Read the model definition and answer for the solid it produces. Units are mm, in the model's axes. A direction names the side the tool comes from. Coordinates: 2 decimals unless noted, no trailing zeros. Write each loop counter-clockwise with the first axis right and the second up, starting at its lowest first coordinate (ties: lowest second). Pieces come first, ordered by that corner, then holes. Notation, with made-up numbers: (11, -10) -> (53, -10) arc R36 ccw to (53, 24) -> close; hole circle Ø5 at (-13, -20). An arc over 180 degrees is marked (long way). One line per item, written item: value. Start each with the question number.
1. For faces 1 (the flat face through (3, -22, -76.2)), 2 (the flat face through (3, -29, 38.1)), 3 (the flat face through (3, 0, 73)), 4 (the flat face through (3, -6, -69.85)), 5 (the flat face through (3, -9, 59.382)), determine the directions among +Z, -Z, +X, -X, +Y, -Y from which every point of the face is accessible in a straight line to the end or side of a thin tool.
2. Find section A-A, the plane y = -4. Write down the section's boundary in (x, z), and give its area (3 significant figures).
3. Find section B-B, the plane z = -2.5. Write down the section's boundary in (x, y), and give its area (3 significant figures).
4. Find section C-C, the plane y = -27.5. Write down the section's boundary in (x, z).
5. Find section D-D, the plane y = 8.5. Write down the section's boundary in (x, z).
6. For a pull along Z with two mould halves and no side action, classify faces 6 (the flat face through (6.35, 10, 1)), 7 (the flat face through (3, 19, 76.2)), 8 (the flat face through (3, -29, -38.1)), 9 (the flat face through (3, -21.293, 3)) as pulls with the +Z half, pulls with the -Z half, needs draft (parallel to the pull), parting line crosses it, or undercut.
7. Given P1, Ø1.9, axis at x = 4, y = 22, coming from the -Z side; P2, Ø3, axis at x = 3, y = 7.5, coming from the +Z side; P3, Ø3, axis at x = 1.5, z = 45, coming from the -Y side, each flat-ended and moving along its own axis, determine where each tip first touches the part or whether it passes through.
8. Consider line 1 along Z through (x, y) = (6.25, -27); line 2 along Z through (x, y) = (3, 21); line 3 along Y through (x, z) = (2.5, 32.5). Determine where each line is inside the solid, lowest interval first.
```python
from build123d import *

# Parameters (mm, degrees)
SKETCH1_W           = 114.3
SKETCH1_H           = 25.4
BOSS_EXTRUDE1_DEPTH = 6.35
SKETCH1_4_W         = 6.35
SKETCH1_4_H         = 6.35
BOSS_EXTRUDE2_DEPTH = 6.35


with BuildPart() as part:
    # Sketch1 → Boss-Extrude1 (new body)
    with BuildSketch(Plane(origin=(0, 0, 0), x_dir=(0, 0, -1), z_dir=(1, 0, 0))):
        Polygon((-76.2, 25.4), (-76.2, 12.7), (-69.85, 12.7), (-69.85, 0), (-76.2, 0), (-76.2, -12.7), (-69.85, -12.7), (-69.85, -31.75), (-63.5, -31.75), (-63.5, -25.4), (-38.1, -25.4), (-38.1, -31.75), (-31.75, -31.75), (-31.75, -25.4), (31.75, -25.4), (31.75, -31.75), (38.1, -31.75), (38.1, -25.4), (63.5, -25.4), (63.5, -31.75), (69.85, -31.75), (69.85, -25.4), (76.2, -25.4), (76.2, -12.7), (69.85, -12.7), (69.85, 0), (76.2, 0), (76.2, 12.7), (69.85, 12.7), (69.85, 25.4), (19.05, 25.4), (19.05, 12.7), (-19.05, 12.7), (-19.05, 25.4), align=None)
        with Locations((-2.231703523, -8.592794364)):
            Rectangle(SKETCH1_W, SKETCH1_H, mode=Mode.SUBTRACT)
    extrude(amount=BOSS_EXTRUDE1_DEPTH)

    # Sketch1<4> → Boss-Extrude2 (add)
    with BuildSketch(Plane(origin=(0, 0, 0), x_dir=(0, 0, -1), z_dir=(1, 0, 0))):
        with Locations((73.025, -28.575)):
            Rectangle(SKETCH1_4_W, SKETCH1_4_H)
    extrude(amount=BOSS_EXTRUDE2_DEPTH)


solid = part.part
```
Answer block:
1. face 1: -Z, +X, -X, +Y, -Y
1. face 2: +X, -X, -Y
1. face 3: +Z, +X, -X
1. face 4: -Z, +X, -X
1. face 5: +X, -X
2. outline: (0, -69.85) -> (6.35, -69.85) -> (6.35, -54.92) -> (0, -54.92) -> close; (0, 59.38) -> (6.35, 59.38) -> (6.35, 76.2) -> (0, 76.2) -> close
2. area: 202 mm2
3. outline: (0, -25.4) -> (6.35, -25.4) -> (6.35, -21.29) -> (0, -21.29) -> close; (0, 4.11) -> (6.35, 4.11) -> (6.35, 12.7) -> (0, 12.7) -> close
3. area: 80.6 mm2
4. outline: (0, -76.2) -> (6.35, -76.2) -> (6.35, -63.5) -> (0, -63.5) -> close; (0, -38.1) -> (6.35, -38.1) -> (6.35, -31.75) -> (0, -31.75) -> close; (0, 31.75) -> (6.35, 31.75) -> (6.35, 38.1) -> (0, 38.1) -> close; (0, 63.5) -> (6.35, 63.5) -> (6.35, 69.85) -> (0, 69.85) -> close
5. outline: (0, -76.2) -> (6.35, -76.2) -> (6.35, 69.85) -> (0, 69.85) -> close
6. face 6: needs draft
6. face 7: pulls with the +Z half
6. face 8: undercut
6. face 9: undercut
7. P1: stops at z = -69.85
7. P2: stops at z = 69.85
7. P3: stops at y = -25.4
8. line 1: z = -76.2 to -63.5, -38.1 to -31.75, 31.75 to 38.1, 63.5 to 69.85
8. line 2: z = -69.85 to -19.05, 19.05 to 76.2
8. line 3: y = -31.75 to -21.29, 4.11 to 25.4
